The model under review builds one solid part; all positions refer to its coordinate system, in mm. Face numbers are marked on the shaded views. A direction names the side the tool comes from. Round coordinates to 2 decimals unless told otherwise and drop trailing zeros. Loops run counter-clockwise (first coordinate to the right, second up) from the corner with the lowest first, then second, coordinate; pieces in that order, holes last. Notation, with made-up numbers: (78, 70.5) -> (111, 70.5) arc R8 cw to (111, 76.5) -> close; hole circle Ø1 at (28, 33). An arc over 180 degrees is marked (long way). Write each question's results on one line, items separated by ' | '. Start each with the question number.
Item 1: We need section B-B (y = 17.5). Give the boundary of the cut face in (x, z), and give its area (3 significant figures).
Item 2: We need section C-C (z = -3.25). Give the number of separate pieces and of enclosed holes in the cut face, and give its area (3 significant figures).
Item 3: Tool access review of the marked faces 1, 2, 3, 4 and 5: name each direction out of +Z, -Z, +X, -X, +Y, -Y from which nothing blocks a thin tool from reaching the whole face with its end or side.
Item 4: We need section D-D (x = 8.5). Give the boundary of the cut face in (y, z).
Item 5: We need section A-A (x = -12.8). Give the boundary of the cut face in (y, z), and give its area (3 significant figures).
Item 6: Clearance check with flat-ended pins moving along their axes: pin 1 Ø8 at (x, y) = (-21.69, 19.3) entering from +Z; pin 2 Ø2 at (x, z) = (-8.5, -2.5) entering from +Y; pin 3 Ø2 at (y, z) = (-7, -4.5) entering from -X; pin 4 Ø4 at (x, y) = (10.5, 1) entering from +Z. State where each tip first meets the part, or that it passes through.
Item 7: Mouldability with a two-part tool opening along Y and no side actions: class the marked faces 6, 7 and 8 as pulls with the +Y half, pulls with the -Y half, needs draft (parallel to the pull), parting line crosses it, or undercut.
Item 8: For L1, parallel to Y at x = -21.5, z = -0.25; L2, parallel to Y at x = 13, z = -2.25; L3, parallel to Y at x = -12.8, z = -5.5, list the stretches that pass through material, from the lowest coordinate up. Write a range as from..to.
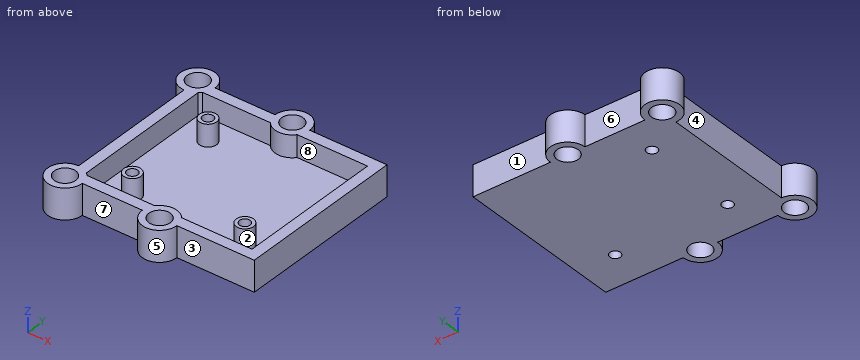
from build123d import *

# Parameters (mm, degrees)
F7_W         = 43.4
F7_H         = 38.6
F8_DEPTH     = 7
F6_W         = 38.4
F6_H         = 33.6
F9_DEPTH     = 7
F10_DEPTH    = 2
F11_R        = 1.9795
F12_DEPTH    = 5
F15_R        = 3.959
F16_DEPTH    = 7
F17_D        = 4.918
F18_D        = 2.459
F18_ON_F11_D = 2.459


with BuildPart() as f8:
    # F7 (on Top) → F8 (new body)
    with BuildSketch(Plane.XY):
        Rectangle(F7_W, F7_H)
    extrude(amount=F8_DEPTH)

    # F6 (on Top) → F9 (cut)
    with BuildSketch(Plane.XY):
        Rectangle(F6_W, F6_H)
    extrude(amount=F9_DEPTH, mode=Mode.SUBTRACT)

    # F6 (on Top) → F10 (join)
    with BuildSketch(Plane.XY):
        Rectangle(F6_W, F6_H)
    extrude(amount=F10_DEPTH)

    # F11 (on face) → F12 (join)
    with BuildSketch(Plane.XY.offset(2)):
        with Locations((-12.8000564873, 10.9999701381)):
            Circle(F11_R)
        with Locations((13.0001017824, -10.9999775887)):
            Circle(F11_R)
        with Locations((-12.8000564873, -10.9999775887)):
            Circle(F11_R)
    extrude(amount=F12_DEPTH)


with BuildPart() as f8_1:
    # F13: moved
    add(f8.part.moved(Location((0, 0, -7))))

    # F15 (on face) → F16 (join)
    with BuildSketch(Plane.XY):
        with Locations((-21.6995608062, -19.3000994623)):
            Circle(F15_R)
        with Locations((0, -19.3000994623)):
            Circle(F15_R)
        with Locations((0, 19.3000193685)):
            Circle(F15_R)
        with Locations((-21.6892641038, 19.3044058979)):
            Circle(F15_R)
    extrude(amount=-F16_DEPTH)

    # F17 (through all)
    with Locations(Plane.XY):
        with Locations((-21.6892641038, 19.3044058979), (0, 19.3000193685), (0, -19.3000994623), (-21.6995608062, -19.3000994623)):
            Hole(F17_D / 2)

    # F18 (through all)
    with Locations(Plane.XY):
        with Locations((-12.8, 11), (13, -11)):
            Hole(F18_D / 2)

    # F18 on F11 (through all)
    with Locations(Plane.XY.offset(2)):
        with Locations((-12.8000564873, -10.9999775887)):
            Hole(F18_ON_F11_D / 2)


solid = f8_1.part
Here are the results:
1) outline: (-25.21, -7) -> (-23.36, -7) -> (-23.36, 0) -> (-25.21, 0) -> close; (-20.02, -7) -> (-1.68, -7) -> (-1.68, 0) -> (-20.02, 0) -> close; (1.68, -7) -> (21.7, -7) -> (21.7, 0) -> (1.68, 0) -> close | area: 282 mm2
2) separate pieces: 4 | enclosed holes: 8 | area: 468 mm2
3) face 1: +Z, -Z, +X, +Y | face 2: +Z | face 3: +Z, -Z, +X, -Y | face 4: +Z, -Z, -X | face 5: +Z, -Z, -Y
4) outline: (-19.3, -7) -> (19.3, -7) -> (19.3, 0) -> (16.8, 0) -> (16.8, -5) -> (-16.8, -5) -> (-16.8, 0) -> (-19.3, 0) -> close
5) outline: (-19.3, -7) -> (-12.23, -7) -> (-12.23, 0) -> (-12.98, 0) -> (-12.98, -5) -> (-16.8, -5) -> (-16.8, 0) -> (-19.3, 0) -> close; (-9.77, -7) -> (9.77, -7) -> (9.77, 0) -> (9.02, 0) -> (9.02, -5) -> (-9.02, -5) -> (-9.02, 0) -> (-9.77, 0) -> close; (12.23, -7) -> (19.3, -7) -> (19.3, 0) -> (16.8, 0) -> (16.8, -5) -> (12.98, -5) -> (12.98, 0) -> (12.23, 0) -> close | area: 107 mm2
6) pin 1: stops at z = 0 | pin 2: stops at y = 19.3 | pin 3: stops at x = -21.7 | pin 4: stops at z = -5
7) face 6: pulls with the +Y half | face 7: pulls with the -Y half | face 8: undercut
8) L1: y = -23.25..-21.75, -16.85..16.85, 21.76..23.26 | L2: y = -19.3..-16.8, -12.98..-12.23, -9.77..-9.02, 16.8..19.3 | L3: y = -19.3..-12.23, -9.77..9.77, 12.23..19.3
